from build123d import *

# Parameters (mm, degrees)
FILLET1_R = 2.54


with BuildPart() as part:
    # Sketch1 → Revolve2 (revolve)
    with BuildSketch(Plane.XY):
        Polygon((-68.58, 0), (68.58, 0), (68.58, 6.35), (38.1, 6.35), (38.1, 15.875), (-38.1, 15.875), (-38.1, 6.35), (-68.58, 6.35), align=None)
    revolve(axis=Axis((-68.58, 0, 0), (1, 0, 0)))

    # Fillet1
    fillet1_edges = [part.edges().sort_by_distance(p)[0] for p in [
        (-68.58, -6.35, 0),
        (68.58, -6.35, 0),
    ]]
    fillet(fillet1_edges, radius=FILLET1_R)


solid = part.part
Work out the finished part from the listing and answer in its coordinate system (mm). A direction names the side the tool comes from. Coordinates: 2 decimals unless noted, no trailing zeros. Write each loop counter-clockwise with the first axis right and the second up, starting at its lowest first coordinate (ties: lowest second). Pieces come first, ordered by that corner, then holes. Notation, with made-up numbers: M -7.75,78.5 L 50.25,78.5 A13 cw 50.25,83.5 Z; hole C 74.5,36.25 d4. An arc over 180 degrees is marked long. Use one line per item in the form item = value. Start each with the question number.
1. A tool of negligible diameter and unlimited length cuts with its end or side. For faces 1 (the face through (-0.533, -3.441, -15.497)), 2 (the face through (-38.1, 7, 0)), 3 (the face through (51.87, -1.38, -6.2)), from which of +Z, -Z, +X, -X, +Y, -Y can it reach the whole face along a straight path? Write none if from no direction.
2. The part is cut by section A-A (z = 0). Give the vertices of the cut face in (x, y) (3 decimals), plus the area to 3 significant figures.
3. Straight lines are drawn through the part: probe 1 along X at (y, z) = (-9.5, -6); probe 2 along Z at (x, y) = (-3, 0) (3 decimals); probe 3 along Y at (x, z) = (-60.5, 0.5). For each, find the intervals that lie inside material, in ascending order. Write a range as from..to.
4. Each of these flat-tipped pins is pushed along its axis until it touches: P1, Ø12, axis at x = -24.5, z = -10.5, coming from the +Y side; P2, Ø4, axis at y = -3.5, z = -7, coming from the +X side; P3, Ø9.5, axis at y = -4.5, z = 7.5, coming from the +X side. Where does it stop, or does it pass through?
5. The part is cut by section D-D (y = -14). Give the vertices of the cut face in (x, z), plus the area to 3 significant figures.
6. The part is cut by section C-C (x = 40). Give the vertices of the cut face in (y, z), plus the area to 3 significant figures.
Evaluation:
q1.face_1 = +X, -X
q1.face_2 = -X
q1.face_3 = +X
q2.outline = M -68.58,-3.81 A2.54 ccw -66.04,-6.35 L -38.1,-6.35 L -38.1,-15.875 L 38.1,-15.875 L 38.1,-6.35 L 66.04,-6.35 A2.54 ccw 68.58,-3.81 L 68.58,3.81 A2.54 ccw 66.04,6.35 L 38.1,6.35 L 38.1,15.875 L -38.1,15.875 L -38.1,6.35 L -66.04,6.35 A2.54 ccw -68.58,3.81 Z
q2.area = 3,190 mm^2
q3.probe_1 = -38.1..38.1
q3.probe_2 = -15.875..15.875
q3.probe_3 = -6.33..6.33
q4.P1 = 15.22
q4.P2 = 67.58
q4.P3 = 68.57
q5.outline = M -38.1,-7.48 L 38.1,-7.48 L 38.1,7.48 L -38.1,7.48 Z
q5.area = 1,140 mm^2
q6.outline = C 0,0 d12.7
q6.area = 127 mm^2
